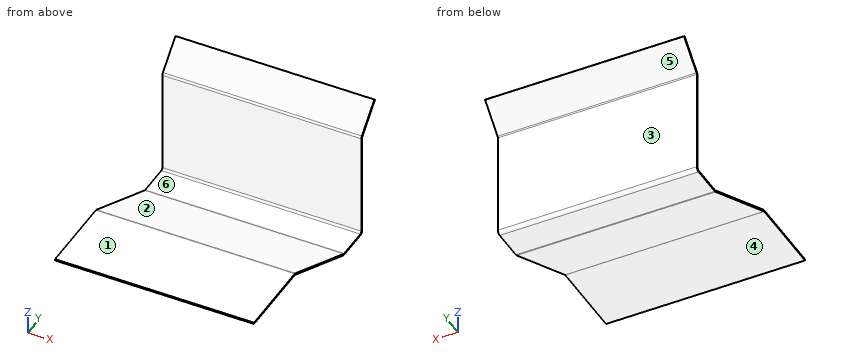
```python
from build123d import *

# Parameters (mm, degrees)
SKETCH1_W          = 200
SKETCH1_H          = 105
BASE_FLANGE1_DEPTH = 1.524
EDGE_FLANGE1_DEPTH = 200
EDGE_FLANGE2_DEPTH = 200
EDGE_FLANGE3_DEPTH = 200
EDGE_FLANGE4_DEPTH = 200


# Sheet-metal steps are written as plain solids
with BuildPart() as part:
    # Sketch1 → Base-Flange1 (new body)
    with BuildSketch(Plane(origin=(0, 0, 0), x_dir=(1, 0, 0), z_dir=(0, 1, 0))):
        Rectangle(SKETCH1_W, SKETCH1_H)
    extrude(amount=-BASE_FLANGE1_DEPTH)

    # Edge-Flange1 section (across the edge) → Edge-Flange1 (add)
    with BuildSketch(Plane(origin=(-100, 0, 53.32063991), x_dir=(0, 0.7071067811865512, -0.7071067811865438), z_dir=(1, 0, 0))):
        with BuildLine():
            Line((-1.524, 0.82063991), (-1.524, 35.368738531))
            Line((-1.524, 35.368738531), (0, 35.368738531))
            Line((0, 35.368738531), (0, 0.82063991))
            ThreePointArc((0, 0.82063991), (0.15080987, 0.062467494), (0.580280045, -0.580280045))
            Line((0.580280045, -0.580280045), (-0.497350689, -1.65791078))
            ThreePointArc((-0.497350689, -1.65791078), (-1.257182537, -0.520742057), (-1.524, 0.82063991))
        make_face()
    extrude(amount=EDGE_FLANGE1_DEPTH)

    # Edge-Flange2 section (across the edge) → Edge-Flange2 (add)
    with BuildSketch(Plane(origin=(-100, -1.524, -54.4812), x_dir=(0, 0, 1), z_dir=(1, 0, 0))):
        with BuildLine():
            Line((-1.524, 1.9812), (-1.524, 33.476))
            Line((-1.524, 33.476), (0, 33.476))
            Line((0, 33.476), (0, 1.9812))
            ThreePointArc((0, 1.9812), (0.580280045, 0.580280045), (1.9812, 0))
            Line((1.9812, 0), (1.9812, -1.524))
            ThreePointArc((1.9812, -1.524), (-0.497350689, -0.497350689), (-1.524, 1.9812))
        make_face()
    extrude(amount=EDGE_FLANGE2_DEPTH)

    # Edge-Flange3 section (across the edge) → Edge-Flange3 (add)
    with BuildSketch(Plane(origin=(-100, -35.439221466, -54.4812), x_dir=(0, 0.4226182617406906, 0.906307787036654), z_dir=(1, 0, 0))):
        with BuildLine():
            Line((-1.524, 0.439221466), (-1.524, 104.662137334))
            Line((-1.524, 104.662137334), (0, 104.662137334))
            Line((0, 104.662137334), (0, 0.439221466))
            ThreePointArc((0, 0.439221466), (0.046962351, 0.010411302), (0.185623012, -0.398069835))
            Line((0.185623012, -0.398069835), (-1.195590055, -1.042140065))
            ThreePointArc((-1.195590055, -1.042140065), (-1.440912764, -0.319442669), (-1.524, 0.439221466))
        make_face()
    extrude(amount=EDGE_FLANGE3_DEPTH)

    # Edge-Flange4 section (across the edge) → Edge-Flange4 (add)
    with BuildSketch(Plane(origin=(100, -131.087402093, -11.561268833), x_dir=(0, 0, -1), z_dir=(-1, 0, 0))):
        with BuildLine():
            Line((-1.524, 0.163300289), (-1.524, 79.662137334))
            Line((-1.524, 79.662137334), (0, 79.662137334))
            Line((0, 79.662137334), (0, 0.163300289))
            ThreePointArc((0, 0.163300289), (0.017460361, 0.003870869), (0.069013684, -0.148000323))
            Line((0.069013684, -0.148000323), (-1.312199383, -0.792070554))
            ThreePointArc((-1.312199383, -0.792070554), (-1.470414754, -0.325983103), (-1.524, 0.163300289))
        make_face()
    extrude(amount=EDGE_FLANGE4_DEPTH)


solid = part.part
```
Verification items for the finished model (mm, model axes). Face numbers are marked on the shaded views. A direction names the side the tool comes from. Give positions to 0.01 mm unless a question says otherwise; leave off trailing zeros. Order: outer loops, then holes, each group sorted by start corner. A loop starts at its lowest first (then second) coordinate and runs counter-clockwise, first axis right, second up. Notation, with made-up numbers: M 59,-12.75 L 116,-12.75 A17 cw 116,12.25 Z; hole C 5.25,-15 d5. An arc over 180 degrees is marked long. Answer in a Markdown table with one row per item. Add a question column.
Item 1: Section check D-D, the plane z = 34. Enter the section's corners in (x, y), and give its area (3 significant figures).
Item 2: Scan lines: probe 1 along Y at (x, z) = (-7, 50.5); probe 2 along Z at (x, y) = (47.5, -11); probe 3 along Y at (x, z) = (38, -16.5). Record each from-to range of solid material in increasing order. Write a range as from..to.
Item 3: Tool access check on the marked faces 4, 5 and 6. Record the directions out of +Z, -Z, +X, -X, +Y, -Y that give a thin tool (end or side, any length) a straight path to the whole face; none if there is none.
Item 4: Section check B-B, the plane z = -21. Enter the section's corners in (x, y).
Item 5: Gauge pin test, flat ends, axial feed: pin 1 (10 mm diameter, centred on x = -27, z = 33, fed in from -Y); pin 2 (2 mm diameter, centred on x = 42.5, y = -75, fed in from +Z); pin 3 (2 mm diameter, centred on x = -32, z = -39.5, fed in from +Y). Record the tip position at first contact, or that the pin passes through.
Item 6: Mould release check, pull along Y, two halves, no side actions. Record for the marked faces 1, 2 and 3: released by +Y, released by -Y, zero draft, split by the parting line, or undercut.
Item 7: Section check A-A, the plane x = 32. Enter the section's corners in (y, z), and give its area (3 significant figures).
Item 8: Section check C-C, the plane y = -173. Enter the section's corners in (x, z), and give its area (3 significant figures).
Filled sheet:
| question | item | result |
|---|---|---|
| 1 | outline | M -100,-1.52 L 100,-1.52 L 100,0 L -100,0 Z |
| 1 | area | 305 mm^2 |
| 2 | probe 1 | y = -1.52..0 |
| 2 | probe 2 | z = -56.01..-54.48 |
| 2 | probe 3 | y = -120.5..-116.89, -1.52..0 |
| 3 | face 4 | -Z, +X, -X, -Y |
| 3 | face 5 | -Z, +X, -X, +Y |
| 3 | face 6 | +Z, +X, -X |
| 4 | outline | M -100,-110.85 L 100,-110.85 L 100,-107.24 L -100,-107.24 Z; M -100,-1.52 L 100,-1.52 L 100,0 L -100,0 Z |
| 5 | pin 1 | stops at y = -1.52 |
| 5 | pin 2 | stops at z = -35.57 |
| 5 | pin 3 | stops at y = 0 |
| 6 | face 1 | zero draft |
| 6 | face 2 | undercut |
| 6 | face 3 | released by +Y |
| 7 | outline | M -210.75,-11.56 L -131.25,-11.56 A0.74 cw -130.94,-11.63 L -36.48,-55.68 A3.51 ccw -35,-56.01 L -3.51,-56.01 A3.51 ccw 0,-52.5 L 0,52.5 A1.98 cw 0.58,53.9 L 25.01,78.33 L 23.93,79.41 L -0.5,54.98 A3.51 ccw -1.52,52.5 L -1.52,-52.5 A1.98 cw -3.51,-54.48 L -35,-54.48 A1.98 cw -35.84,-54.3 L -130.3,-10.25 A2.26 ccw -131.25,-10.04 L -210.75,-10.04 Z |
| 7 | area | 553 mm^2 |
| 8 | outline | M -100,-11.56 L 100,-11.56 L 100,-10.04 L -100,-10.04 Z |
| 8 | area | 305 mm^2 |
